Here's how the part is built. I have some questions about the finished solid (model axes, mm). A direction names the side the tool comes from. Round coordinates to 2 decimals unless told otherwise and drop trailing zeros. Loops run counter-clockwise (first coordinate to the right, second up) from the corner with the lowest first, then second, coordinate; pieces in that order, holes last. Notation, with made-up numbers: M -27,74 L 24,74 A24 cw 24,106 Z; hole C 67,14.5 d9. An arc over 180 degrees is marked long. Put each result on its own line as item: value. Start each with the question number.
```python
from build123d import *

# Parameters (mm, degrees)
F1_DEPTH = 5
F2_R     = 5
F3_DEPTH = 10
F4_R     = 5
F5_DEPTH = 15


with BuildPart() as f1:
    # F0 (on Top) → F1 (new body)
    with BuildSketch(Plane.XY):
        with BuildLine():
            ThreePointArc((0, 20), (-10, 10), (0, 0))
            Line((0, 0), (30, 0))
            ThreePointArc((30, 0), (40, 10), (30, 20))
            Line((30, 20), (0, 20))
        make_face()
    extrude(amount=F1_DEPTH)

    # F2 (on Top) → F3 (join)
    with BuildSketch(Plane.XY):
        with Locations((0, 10)):
            Circle(F2_R)
    extrude(amount=-F3_DEPTH)

    # F4 (on Top) → F5 (join)
    with BuildSketch(Plane.XY):
        with Locations((30, 10)):
            Circle(F4_R)
    extrude(amount=F5_DEPTH)


solid = f1.part
```
1) Suppose I cut it at A-A (x = 32). Write out the boundary of the cut face in (y, z).
2) On a 3-axis mill with a long thin cutter (end or side, diameter ignored), from which of +Z, -Z, +X, -X, +Y, -Y can I reach the whole of each face in a straight line? I mean faces 1 (the face through (-10, 10, 2)), 2 (the face through (-0.651, 14.957, -4.93)), 3 (the face through (25, 10, 10)). Say none if no direction works.
3) Suppose I cut it at C-C (z = -1.75). Write out the boundary of the cut face in (x, y), plus the area to 3 significant figures.
4) Suppose I cut it at D-D (y = 2). Write out the boundary of the cut face in (x, z).
5) I'm going to push flat-ended pins straight in: P1, Ø3, axis at x = 19, y = 13.5, coming from the -Z side; P2, Ø1.5, axis at y = 7.5, z = -6.5, coming from the +X side; P3, Ø10, axis at y = 16.5, z = 6.5, coming from the +X side; P4, Ø6, axis at x = 6, y = 14.5, coming from the -Z side. Where does each tip first touch, or does it pass through?
6) If I drill on probe 1 along Z at (x, y) = (20, 18.5); probe 2 along Z at (x, y) = (-4, 9.25); probe 3 along X at (y, z) = (13, 5.5), over which ranges is the centre line in solid material (lowest first)? Write a range as from..to.
7) Suppose I cut it at B-B (y = 10). Write out the boundary of the cut face in (x, z).
Results are:
1. outline: M 0.2,0 L 19.8,0 L 19.8,5 L 14.58,5 L 14.58,15 L 5.42,15 L 5.42,5 L 0.2,5 Z
2. face 1: +Z, -Z, -X
2. face 2: -Z
2. face 3: +Z
3. outline: C 0,10 d10
3. area: 78.5 mm²
4. outline: M -6,0 L 36,0 L 36,5 L -6,5 Z
5. P1: z = 0
5. P2: x = 4.68
5. P3: x = 39.85
5. P4: z = -10
6. probe 1: 0..5
6. probe 2: -10..5
6. probe 3: 26..34
7. outline: M -10,0 L -5,0 L -5,-10 L 5,-10 L 5,0 L 40,0 L 40,5 L 35,5 L 35,15 L 25,15 L 25,5 L -10,5 Z
